Geometry: final body of the model. Coordinates: model frame, mm. A direction names the side the tool comes from. Give positions to 0.01 mm unless a question says otherwise; leave off trailing zeros. Write each loop counter-clockwise with the first axis right and the second up, starting at its lowest first coordinate (ties: lowest second). Pieces come first, ordered by that corner, then holes. Notation, with made-up numbers: (5, -10.5) - (50, -10.5) arc R20 ccw to (50, 12.5) - close; hole circle Ø9 at (15, 1.25). An arc over 180 degrees is marked (long way). Return JSON: item names as keys, results as strings.
Autodesk Inventor part; units mm, degrees
ref_plane "YZ Plane" through (0, 0, 0) normal (1, 0, 0) x (0, 1, 0)
ref_plane "XZ Plane" through (0, 0, 0) normal (0, 1, 0) x (-1, 0, 0)
ref_plane "XY Plane" through (0, 0, 0) normal (0, 0, 1) x (1, 0, 0)
sketch "スケッチ1" plane through (0, 0, 0) normal (1, 0, 0) x (0, 1, 0)
  line L0 (0, 0) -> (9, 0)
  line L1 (9, 0) -> (9, -9)
  line L2 (9, -9) -> (0, -9)
  line L3 (0, -9) -> (0, 0)
  line L4 (1.2, -1.2) -> (7.8, -1.2)
  line L5 (7.8, -1.2) -> (7.8, -7.8)
  line L6 (7.8, -7.8) -> (1.2, -7.8)
  line L7 (1.2, -7.8) -> (1.2, -1.2)
  dimension "d0" = 9
  dimension "d1" = 9
  dimension "d2" = 1.2
  dimension "d3" = 1.2
  dimension "d4" = 1.2
  dimension "d5" = 1.2
extrude "押し出し1" add sketch "スケッチ1" along normal blind 99.5097
sketch "スケッチ2" plane through (0, 0, -9) normal (0, -1, 0) x (1, 0, 0)
  line L0 (0, 9) -> (0, 0)
  line L1 (99.5097, 9) -> (99.5097, 0)
  line L2 (0, 9) -> (99.5097, 9)
  point P0 (95.0097, 4.5)
  point P1 (4.5, 4.5)
  dimension "d8" = 4.5
  dimension "d9" = 4.5
  dimension "d10" = 4.5
  dimension "d11" = 4.5
hole "穴1" at (95.0097, 0, -4.5) at (4.5, 0, -4.5) direction (0, 1, 0) diameter 5 end through all
sketch "スケッチ3" plane through (0, 0, 0) normal (0, 0, 1) x (1, 0, 0)
  line L0 (0, 9) -> (0, 0)
  line L1 (0, 9) -> (99.5097, 9)
  line L2 (99.5097, 9) -> (99.5097, 0)
  point P0 (13.5, 4.5)
  point P1 (86.0097, 4.5)
  dimension "d19" = 13.5
  dimension "d20" = 4.5
  dimension "d21" = 4.5
  dimension "d22" = 13.5
hole "穴2" at (13.5, 4.5, 0) at (86.0097, 4.5, 0) direction (0, 0, -1) diameter 3 end through all
sketch "スケッチ5" plane through (0, 0, -9) normal (0, 0, -1) x (-1, 0, 0)
  line L0 (-99.5097, 0) -> (-99.5097, 9)
  line L1 (0, 9) -> (-99.5097, 9)
  point P0 (0, 0)
  point P1 (-21.0097, 4.5)
  dimension "d39" = 78.5
  dimension "d40" = 4.5
hole "穴4" at (21.0097, 4.5, -9) direction (0, 0, 1) diameter 3 end through all
sketch "スケッチ6" plane through (0, 0, -9) normal (0, -1, 0) x (1, 0, 0)
  circle A0 centre (95.0097, 4.5) radius 2.5
  circle A1 centre (4.5, 4.5) radius 2.5
  line L0 (4.5, 4.5) -> (95.0097, 4.5)
  point P0 (0, 9)
  point P1 (88.5447, 4.5)
  point P2 (82.0797, 4.5)
  point P3 (75.6147, 4.5)
  point P4 (69.1498, 4.5)
  point P5 (62.6848, 4.5)
  point P6 (56.2198, 4.5)
  point P7 (49.7548, 4.5)
  point P8 (43.2899, 4.5)
  point P9 (36.8249, 4.5)
  point P10 (30.3599, 4.5)
  point P11 (23.8949, 4.5)
  point P12 (17.43, 4.5)
  point P13 (10.965, 4.5)
  dimension "d48" = 90.5097
  dimension "d49" = 6.465
  dimension "d52" = 6.465
hole "穴5" at (88.5447, 0, -4.5) at (82.0797, 0, -4.5) at (75.6147, 0, -4.5) at (69.1498, 0, -4.5) at (62.6848, 0, -4.5) at (56.2198, 0, -4.5) at (49.7548, 0, -4.5) at (43.2899, 0, -4.5) at (36.8249, 0, -4.5) at (30.3599, 0, -4.5) at (23.8949, 0, -4.5) at (17.43, 0, -4.5) at (10.965, 0, -4.5) direction (0, 1, 0) diameter 5.5 end through all
sketch "スケッチ7" plane through (0, 0, -9) normal (0, 0, -1) x (-1, 0, 0)
  line L0 (0, 9) -> (-99.5097, 9)
  circle A0 centre (-13.5, 4.5) radius 1.5
  line L1 (0, 0) -> (0, 9)
  line L2 (-99.5097, 0) -> (-99.5097, 9)
  circle A1 centre (-86.0097, 4.5) radius 1.5
  circle A2 centre (-21.0097, 4.5) radius 1.5
  line L3 (-86.0097, 4.5) -> (-21.0097, 4.5)
  point P0 (-92.7597, 4.5)
  point P1 (-6.75, 4.5)
  point P2 (-79.5097, 4.5)
  point P3 (-73.0097, 4.5)
  point P4 (-66.5097, 4.5)
  point P5 (-60.0097, 4.5)
  point P6 (-53.5097, 4.5)
  point P7 (-47.0097, 4.5)
  point P8 (-40.5097, 4.5)
  point P9 (-34.0097, 4.5)
  point P10 (-27.5097, 4.5)
  dimension "d64" = 4.5
  dimension "d65" = 4.5
  dimension "d68" = 13.5
  dimension "d69" = 6.75
  dimension "d70" = 13.5
  dimension "d71" = 6.75
  dimension "d72" = 65
  dimension "d73" = 6.5
  dimension "d76" = 6.5
hole "穴6" at (92.7597, 4.5, -9) at (6.75, 4.5, -9) at (79.5097, 4.5, -9) at (73.0097, 4.5, -9) at (66.5097, 4.5, -9) at (60.0097, 4.5, -9) at (53.5097, 4.5, -9) at (47.0097, 4.5, -9) at (40.5097, 4.5, -9) at (34.0097, 4.5, -9) at (27.5097, 4.5, -9) direction (0, 0, 1) diameter 5.5 end through all
equation "\"d3\" = d2"
equation "\"d4\" = d2"
equation "\"d5\" = d4"
properties part number "ロボット回転9ｘ9_1" material "アルミニウム 6061"
Q1. Section query C-C, the plane z = -4.5. Count the separate pieces of the cut face and the enclosed holes in it, plus the area to 3 significant figures.
Answer key:
{"separate pieces": "32", "enclosed holes": "0", "area": "43.2 mm^2"}
Q2. Mould query, pull axis Y, two halves, no side actions, for faces 3 (the cylindrical face through (95.444, 3.904, -8.392)), 4 (the cylindrical face through (45.975, 8.408, -3.904)). Classes: pulls with the +Y half, pulls with the -Y half, needs draft (parallel to the pull), parting line crosses it, or undercut.
Answer key:
{"face 3": "undercut", "face 4": "needs draft"}
Q3. Material intervals for probe 1 along Z at (x, y) = (90, 3.5); probe 2 along Y at (x, z) = (12.5, -7); probe 3 along Z at (x, y) = (43.5, 0.5), sorted ascending. Write a range as [from, to].
Answer key:
{"probe 1": "z = [-9, -7.8], [-1.2, 0]", "probe 2": "y = [0, 1.2], [7.8, 9]", "probe 3": "z = [-9, -7.24], [-1.76, 0]"}
Q4. Section query A-A, the plane x = 17.43. Return the cut outline in (y, z).
Answer key:
{"outline": "(0, -9) - (9, -9) - (9, -7.25) - (7.8, -7.25) - (7.8, -7.8) - (1.2, -7.8) - (1.2, -7.25) - (0, -7.25) - close; (0, -1.75) - (1.2, -1.75) - (1.2, -1.2) - (7.8, -1.2) - (7.8, -1.75) - (9, -1.75) - (9, 0) - (0, 0) - close"}
Q5. Section query B-B, the plane x = 48. Return the cut outline in (y, z), plus the area to 3 significant figures.
Answer key:
{"outline": "(0, -9) - (1.93, -9) - (1.93, -7.8) - (1.2, -7.8) - (1.2, -6.62) - (0, -6.62) - close; (0, -2.38) - (1.2, -2.38) - (1.2, -1.2) - (1.93, -1.2) - (1.93, 0) - (0, 0) - close; (7.07, -9) - (9, -9) - (9, -6.62) - (7.8, -6.62) - (7.8, -7.8) - (7.07, -7.8) - close; (7.07, -1.2) - (7.8, -1.2) - (7.8, -2.38) - (9, -2.38) - (9, 0) - (7.07, 0) - close", "area": "15.0 mm^2"}
Q6. Set-up query: faces 1 (the cylindrical face through (66.423, 8.408, -4.142)), 2 (the flat face through (49, 7, -7.8)). Return all of +Z, -Z, +X, -X, +Y, -Y with unobstructed straight access to the full face (end or side cutting, diameter ignored); none if empty.
Answer key:
{"face 1": "+Y, -Y", "face 2": "+X, -X"}
